```python
from build123d import *

# Parameters (mm, degrees)
SKETCH1_W           = 75
SKETCH1_H           = 3
BOSS_EXTRUDE1_DEPTH = 200
SKETCH2_R           = 4.9
BOSS_EXTRUDE2_DEPTH = 10
SKETCH3_W           = 7
SKETCH3_H           = 33
SKETCH3_W_2         = 5
SKETCH3_H_2         = 30
CUT_EXTRUDE1_DEPTH  = 1


with BuildPart() as part:
    # Sketch1 → Boss-Extrude1 (new body)
    with BuildSketch(Plane.XY):
        with Locations((37.5, 1.5)):
            Rectangle(SKETCH1_W, SKETCH1_H)
    extrude(amount=BOSS_EXTRUDE1_DEPTH)

    # Sketch2 → Boss-Extrude2 (add)
    with BuildSketch(Plane(origin=(0, 3, 0), x_dir=(1, 0, 0), z_dir=(0, 1, 0))):
        with Locations(Location((12.5, -10, 0), (0, 0, 90))):
            Circle(SKETCH2_R)
        with Locations(Location((52.5, -190, 0), (0, 0, 90))):
            Circle(SKETCH2_R)
    extrude(amount=BOSS_EXTRUDE2_DEPTH)

    # Sketch3 → Cut-Extrude1 (cut)
    with BuildSketch(Plane.XZ):
        with Locations((7.5, 26.5)):
            Rectangle(SKETCH3_W, SKETCH3_H)
        with Locations((7.5, 63.5)):
            Rectangle(SKETCH3_W, SKETCH3_H)
        with Locations((27.5, 135)):
            Rectangle(SKETCH3_W_2, SKETCH3_H_2)
        with Locations((22.5, 26.5)):
            Rectangle(SKETCH3_W, SKETCH3_H)
        with Locations((22.5, 63.5)):
            Rectangle(SKETCH3_W, SKETCH3_H)
        with Locations((37.5, 26.5)):
            Rectangle(SKETCH3_W, SKETCH3_H)
        with Locations((37.5, 63.5)):
            Rectangle(SKETCH3_W, SKETCH3_H)
        with Locations((52.5, 26.5)):
            Rectangle(SKETCH3_W, SKETCH3_H)
        with Locations((52.5, 63.5)):
            Rectangle(SKETCH3_W, SKETCH3_H)
        with Locations((67.5, 26.5)):
            Rectangle(SKETCH3_W, SKETCH3_H)
        with Locations((67.5, 63.5)):
            Rectangle(SKETCH3_W, SKETCH3_H)
        with Locations((27.5, 185)):
            Rectangle(SKETCH3_W_2, SKETCH3_H_2)
    extrude(amount=-CUT_EXTRUDE1_DEPTH, mode=Mode.SUBTRACT)


solid = part.part
```
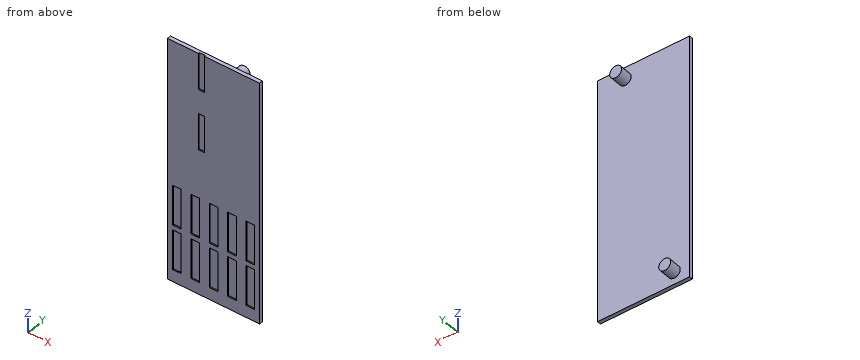
The listing builds one solid part. Answer for the finished solid, in the listing's coordinates (mm). Give positions to 0.01 mm unless a question says otherwise; leave off trailing zeros. Write each loop counter-clockwise with the first axis right and the second up, starting at its lowest first coordinate (ties: lowest second). Pieces come first, ordered by that corner, then holes. Notation, with made-up numbers: (65.25, 87) - (120.25, 87) arc R12 ccw to (120.25, 110) - close; hole circle Ø3 at (31, -7). An arc over 180 degrees is marked (long way). Use one line per item in the form item = value. Start each with the question number.
1) Find section B-B on z = 17.5. Determine the outline of the cut face in (x, y), plus the area to 3 significant figures.
2) Find section C-C on y = 5. Determine the outline of the cut face in (x, z), plus the area to 3 significant figures.
3) Find section D-D on z = 190. Determine the outline of the cut face in (x, y).
4) Find section A-A on x = 52.5. Determine the outline of the cut face in (y, z).
5) Flat-ended cylindrical pins translate along their axes: pin 1 Ø5 at (x, y) = (10, 8) entering from +Z; pin 2 Ø0.8 at (x, y) = (27.5, 0.5) entering from +Z; pin 3 Ø5 at (x, y) = (60.5, 11) entering from -Z; pin 4 Ø8 at (x, z) = (8, 33) entering from +Y. Find the tip coordinate at first contact, or state that the pin passes through.
6) Consider line 1 along Y through (x, z) = (32, 21); line 2 along Y through (x, z) = (25, 40); line 3 along Z through (x, y) = (52.5, 10.25). Determine where each line is inside the solid, lowest interval first. Write a range as from..to.
Geometry results:
q1.outline = (0, 0) - (4, 0) - (4, 1) - (11, 1) - (11, 0) - (19, 0) - (19, 1) - (26, 1) - (26, 0) - (34, 0) - (34, 1) - (41, 1) - (41, 0) - (49, 0) - (49, 1) - (56, 1) - (56, 0) - (64, 0) - (64, 1) - (71, 1) - (71, 0) - (75, 0) - (75, 3) - (0, 3) - close
q1.area = 190 mm2
q2.outline = circle Ø9.8 at (12.5, 10); circle Ø9.8 at (52.5, 190)
q2.area = 151 mm2
q3.outline = (0, 0) - (25, 0) - (25, 1) - (30, 1) - (30, 0) - (75, 0) - (75, 3) - (57.4, 3) - (57.4, 13) - (47.6, 13) - (47.6, 3) - (0, 3) - close
q4.outline = (0, 0) - (3, 0) - (3, 185.1) - (13, 185.1) - (13, 194.9) - (3, 194.9) - (3, 200) - (0, 200) - (0, 80) - (1, 80) - (1, 47) - (0, 47) - (0, 43) - (1, 43) - (1, 10) - (0, 10) - close
q5.pin_1 = 14.9
q5.pin_2 = 170
q5.pin_3 = through
q5.pin_4 = 3
q6.line_1 = 0..3
q6.line_2 = 1..3
q6.line_3 = 185.1..194.9
